```python
from build123d import *

# Parameters (mm, degrees)
F2_SIZE  = 2.54
F5_DEPTH = 22.86
F4_R     = 5.969
F6_DEPTH = 176.3532


with BuildPart() as f1:
    # F0 (on Front) → F1 (revolve)
    with BuildSketch(Plane.XZ):
        Polygon((15.5575, 0), (20.6375, 0), (20.6375, 24.765), (28.6639, 24.765), (28.6639, 32.385), (53.975, 43.18), (81.28, 43.18), (81.28, 51.1048), (57.15, 51.1048), (57.15, 58.7248), (55.88, 58.7248), (55.88, 146.869346), (26.9875, 180.7972), (20.6375, 180.7972), (20.6375, 201.1172), (15.5575, 201.1172), align=None)
    revolve(axis=Axis((0, 0, 0.880979), (0, 0, -1)))

    # F2
    f2_edges = [f1.edges().sort_by_distance(p)[0] for p in [
        (-15.5575, 0, 201.1172),
        (-15.5575, 0, 0),
        (15.5575, 0, 100.5586),
    ]]
    chamfer(f2_edges, length=F2_SIZE)

    # F4 (on offset) → F5 (cut)
    with BuildSketch(Plane(origin=(0, 0, 24.765), x_dir=(1, 0, 0), z_dir=(0, 0, -1))):
        with BuildLine():
            ThreePointArc((17.438577, 23.688146), (25.47399, 14.707415), (29.233824, 3.258178))
            Line((29.233824, 3.258178), (55.293112, 3.258178))
            ThreePointArc((55.293112, 3.258178), (47.968302, 27.694512), (30.468221, 46.256151))
            Line((30.468221, 46.256151), (17.438577, 23.688146))
        make_face()
        with BuildLine():
            ThreePointArc((-11.795247, 26.946324), (0, 29.41483), (11.795247, 26.946324))
            Line((11.795247, 26.946324), (24.824891, 49.514329))
            ThreePointArc((24.824891, 49.514329), (0, 55.389024), (-24.824891, 49.514329))
            Line((-24.824891, 49.514329), (-11.795247, 26.946324))
        make_face()
        with BuildLine():
            ThreePointArc((-29.233824, 3.258178), (-25.47399, 14.707415), (-17.438577, 23.688146))
            Line((-17.438577, 23.688146), (-30.468221, 46.256151))
            ThreePointArc((-30.468221, 46.256151), (-47.968302, 27.694512), (-55.293112, 3.258178))
            Line((-55.293112, 3.258178), (-29.233824, 3.258178))
        make_face()
        with BuildLine():
            Line((-30.468221, -46.256151), (-17.438577, -23.688146))
            ThreePointArc((-17.438577, -23.688146), (-25.47399, -14.707415), (-29.233824, -3.258178))
            Line((-29.233824, -3.258178), (-55.293112, -3.258178))
            ThreePointArc((-55.293112, -3.258178), (-47.968302, -27.694512), (-30.468221, -46.256151))
        make_face()
        with BuildLine():
            Line((24.824891, -49.514329), (11.795247, -26.946324))
            ThreePointArc((11.795247, -26.946324), (0, -29.41483), (-11.795247, -26.946324))
            Line((-11.795247, -26.946324), (-24.824891, -49.514329))
            ThreePointArc((-24.824891, -49.514329), (0, -55.389024), (24.824891, -49.514329))
        make_face()
        with BuildLine():
            Line((55.293112, -3.258178), (29.233824, -3.258178))
            ThreePointArc((29.233824, -3.258178), (25.47399, -14.707415), (17.438577, -23.688146))
            Line((17.438577, -23.688146), (30.468221, -46.256151))
            ThreePointArc((30.468221, -46.256151), (47.968302, -27.694512), (55.293112, -3.258178))
        make_face()
    extrude(amount=-F5_DEPTH, mode=Mode.SUBTRACT)

    # F4 (on offset) → F6 (cut, through all)
    with BuildSketch(Plane(origin=(0, 0, 24.765), x_dir=(1, 0, 0), z_dir=(0, 0, -1))):
        with Locations((0, 69.9897)):
            Circle(F4_R)
        with Locations((41.138913, 56.622857)):
            Circle(F4_R)
        with Locations((66.56416, 21.628007)):
            Circle(F4_R)
        with Locations((66.56416, -21.628007)):
            Circle(F4_R)
        with Locations((-41.138913, 56.622857)):
            Circle(F4_R)
        with Locations((-66.56416, 21.628007)):
            Circle(F4_R)
        with Locations((-66.56416, -21.628007)):
            Circle(F4_R)
        with Locations((-41.138913, -56.622857)):
            Circle(F4_R)
        with Locations((0, -69.9897)):
            Circle(F4_R)
        with Locations((41.138913, -56.622857)):
            Circle(F4_R)
    extrude(amount=-F6_DEPTH, mode=Mode.SUBTRACT)


solid = f1.part
```
Here's how the part is built. I have some questions about the finished solid (model axes, mm). A direction names the side the tool comes from. Give positions to 0.01 mm unless a question says otherwise; leave off trailing zeros. Loops run counter-clockwise (first coordinate to the right, second up) from the corner with the lowest first, then second, coordinate; pieces in that order, holes last. Notation, with made-up numbers: (34.25, 23.5) -> (84.25, 23.5) arc R23 cw to (84.25, 55.5) -> close; hole circle Ø5 at (22, 71). An arc over 180 degrees is marked (long way). Use one line per item in the form item = value. Start each with the question number.
1) Which directions (+Z, -Z, +X, -X, +Y, -Y) give clear straight access to the entire face, cutting with the end or side of a thin tool? Please do faces 4 (the face through (-0.17, -29.414, 40.061)), 5 (the face through (-10.58, -80.59, 47.2)), 6 (the face through (-57.095, -2.513, 54.968)).
2) Thinking about a two-plate mould opening in Y: for faces 1 (the face through (-7.3, -55.4, 103.4)), 2 (the face through (-0.36, 55.388, 45.371)), 3 (the face through (20, -7, 24.765)), which applies, +Y half, -Y half, draft (parallel to the pull), parting line (faces both ways), or undercut?
3) Imagine slicing it at B-B (x = 0). Count the separate pieces of the cut face and the enclosed holes in it, then the cut area to 3 significant figures.
4) Imagine slicing it at A-A (z = 187.5). Please give me the cut outline in (x, y) (1 decimal), then the cut area to 3 significant figures.
5) For P1, Ø12, axis at x = -39.5, z = 22, coming from the -Y side; P2, Ø15.5, axis at x = -41.14, y = 56.62, coming from the -Z side; P3, Ø10, axis at y = -2.5, z = 66, coming from the -X side; P4, Ø6, axis at y = -39, z = 164.5, coming from the -X side, each with a flat end and sliding along its axis, tell me the tip position at first contact or that it passes through.
6) Please list where these lines run through material, in increasing order: line 1 along Y through (x, z) = (0, 46.5); line 2 along Z through (x, y) = (-38.5, 47); line 3 along Y through (x, z) = (-26.5, 56).
Check values:
q1.face_4 = -Z
q1.face_5 = +Z, -Z
q1.face_6 = +Z
q2.face_1 = parting line
q2.face_2 = undercut
q2.face_3 = draft
q3.separate_pieces = 4
q3.enclosed_holes = 0
q3.area = 11,100 mm^2
q4.outline = circle Ø41.3 at (0, 0); hole circle Ø31.1 at (0, 0)
q4.area = 578 mm^2
q5.P1 = through
q5.P2 = 43.18
q5.P3 = -55.88
q5.P4 = -21.47
q6.line_1 = -81.28 to -75.96, -64.02 to -55.39, -29.41 to -15.56, 15.56 to 29.41, 55.39 to 64.02, 75.96 to 81.28
q6.line_2 = 43.18 to 51.1
q6.line_3 = -50.63 to 50.63
